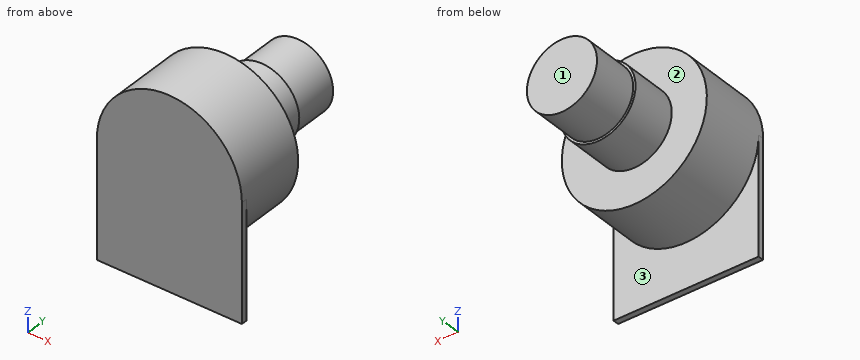
from build123d import *

# Parameters (mm, degrees)
SKETCH_1_R      = 6.2
EXTRUDE_1_DEPTH = 6.22
EXTRUDE_2_DEPTH = 0.5
SKETCH_3_R      = 3.2
EXTRUDE_3_DEPTH = 4
SKETCH_4_R      = 3
EXTRUDE_4_DEPTH = 4


with BuildPart() as part:
    # Эскиз1 → Вытянуть1 (new body)
    with BuildSketch(Plane(origin=(0, 0, 0), x_dir=(1, 0, 0), z_dir=(0, 1, 0))):
        with Locations(Location((0, 0, 0), (0, 0, 270))):
            Circle(SKETCH_1_R)
    extrude(amount=EXTRUDE_1_DEPTH)

    # Эскиз2 → Вытянуть2 (add)
    with BuildSketch(Plane.XZ):
        with BuildLine():
            Line((-6.2, 0), (-6.2, -10))
            Line((-6.2, -10), (6.2, -10))
            Line((6.2, -10), (6.2, 0))
            ThreePointArc((6.2, 0), (0, 6.2), (-6.2, 0))
        make_face()
    extrude(amount=-EXTRUDE_2_DEPTH)

    # Эскиз3 → Вытянуть3 (add)
    with BuildSketch(Plane(origin=(0, 6.22, 0), x_dir=(1, 0, 0), z_dir=(0, 1, 0))):
        with Locations(Location((0, 0, 0), (0, 0, 270))):
            Circle(SKETCH_3_R)
    extrude(amount=EXTRUDE_3_DEPTH)

    # Эскиз4 → Вытянуть4 (add)
    with BuildSketch(Plane(origin=(0, 10.22, 0), x_dir=(-1, 0, 0), z_dir=(0, 1, 0))):
        with Locations(Location((0, 0, 0), (0, 0, 90))):
            Circle(SKETCH_4_R)
    extrude(amount=EXTRUDE_4_DEPTH)


solid = part.part
Build history of the part. All positions in model axes, mm. Face numbers are marked on the shaded views. A direction names the side the tool comes from. Give positions to 0.01 mm unless a question says otherwise; leave off trailing zeros. Order: outer loops, then holes, each group sorted by start corner. A loop starts at its lowest first (then second) coordinate and runs counter-clockwise, first axis right, second up. Notation, with made-up numbers: M -4,70 L 22,70 A20 ccw 22,95 Z; hole C -32.5,-25.5 d7. An arc over 180 degrees is marked long. Put each result on its own line as item: value.
Item 1: Cut at A-A on x = 0. Write the cut outline in (y, z).
Results are:
outline: M 0,-10 L 0.5,-10 L 0.5,-6.2 L 6.22,-6.2 L 6.22,-3.2 L 10.22,-3.2 L 10.22,-3 L 14.22,-3 L 14.22,3 L 10.22,3 L 10.22,3.2 L 6.22,3.2 L 6.22,6.2 L 0,6.2 Z
Item 2: Drop flat-ended pins along their axis: pin 1 Ø4 at (x, y) = (-4.5, 10.5) entering from +Z; pin 2 Ø2 at (y, z) = (6.5, -3) entering from +X; pin 3 Ø2 at (y, z) = (3.5, -4.5) entering from -X. Give the stop position or say it passes through.
Results are:
pin 1: z = 1.97
pin 2: x = 5.85
pin 3: x = -5.12
Item 3: Cut at B-B on z = 0.25. Write the cut outline in (x, y), then the cut area to 3 significant figures.
Results are:
outline: M -6.19,0 L 6.19,0 L 6.19,6.22 L 3.19,6.22 L 3.19,10.22 L 2.99,10.22 L 2.99,14.22 L -2.99,14.22 L -2.99,10.22 L -3.19,10.22 L -3.19,6.22 L -6.19,6.22 Z
area: 127 mm2
Item 4: Cut at C-C on y = 9.75. Write the cut outline in (x, z).
Results are:
outline: C 0,0 d6.4
Item 5: Which spindle directions (+Z, -Z, +X, -X, +Y, -Y) get a long thin tool onto all of the face, cutting with end or side? Do the marked faces 1, 2 and 3. Say none if no direction does.
Results are:
face 1: +Z, -Z, +X, -X, +Y
face 2: +Y
face 3: -Z, +Y
Item 6: Wall check: probe 1 along Z at (x, y) = (0, 5.5); probe 2 along Y at (x, z) = (3, -7.75); probe 3 along Y at (x, z) = (-3.25, 2.75). Give the ranges that are in metal, low to high.
Results are:
probe 1: -6.2 to 6.2
probe 2: 0 to 0.5
probe 3: 0 to 6.22
Item 7: Cut at D-D on z = -2. Write the cut outline in (x, y).
Results are:
outline: M -6.2,0 L 6.2,0 L 6.2,0.5 L 5.87,0.5 L 5.87,6.22 L 2.5,6.22 L 2.5,10.22 L 2.24,10.22 L 2.24,14.22 L -2.24,14.22 L -2.24,10.22 L -2.5,10.22 L -2.5,6.22 L -5.87,6.22 L -5.87,0.5 L -6.2,0.5 Z
